Autodesk Inventor part; units mm, degrees
ref_plane "YZ Plane" through (0, 0, 0) normal (1, 0, 0) x (0, 1, 0)
ref_plane "XZ Plane" through (0, 0, 0) normal (0, 1, 0) x (-1, 0, 0)
ref_plane "XY Plane" through (0, 0, 0) normal (0, 0, 1) x (1, 0, 0)
sketch "Sketch1" plane through (0, 0, 0) normal (0, 1, 0) x (-1, 0, 0)
  circle A0 centre (0, 0) radius 30
  circle A1 centre (0, 0) radius 8.5
  dimension "d0" = 60
  dimension "d1" = 17
extrude "Extrusion1" add sketch "Sketch1" along normal blind 30
sketch "Sketch2" plane through (0, 30, 0) normal (0, 1, 0) x (1, 0, 0)
  circle A0 centre (0, 0) radius 21
  dimension "d4" = 42
extrude "Extrusion2" cut sketch "Sketch2" against normal blind 20
fillet "Fillet1" radius 2 1 edges at (30, 30, 0)
fillet "Fillet2" radius 0.5 1 edges at (-21, 30, 0)
shell "Shell2" thickness 1.5 removed faces 1 at (-22.4604, 0, -3.0712)
properties part number "FrontWheel"
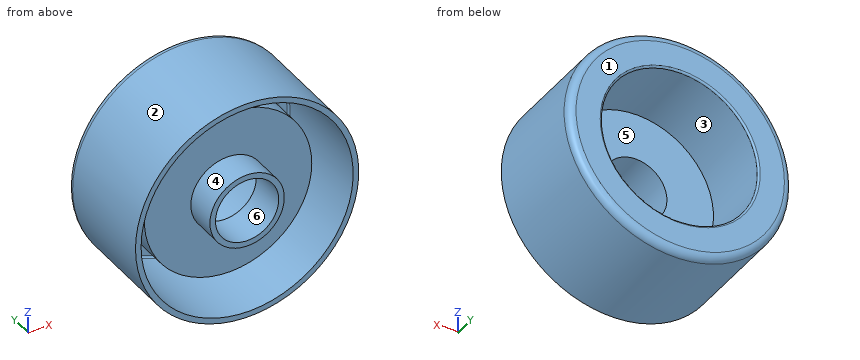
The listing builds one solid part. Answer for the finished solid, in the listing's coordinates (mm). Face numbers are marked on the shaded views. A direction names the side the tool comes from. Coordinates: 2 decimals unless noted, no trailing zeros. Order: outer loops, then holes, each group sorted by start corner. A loop starts at its lowest first (then second) coordinate and runs counter-clockwise, first axis right, second up. Notation, with made-up numbers: M -23.5,-4 L 14.5,-4 A25 cw 14.5,18 Z; hole C 6,-40 d10. An arc over 180 degrees is marked long. Use CSV: the item, a comma, the result in double quotes.
Q1. Determine the mould class of the marked faces 1, 2 and 3 for opening direction X: pulls with the +X half, pulls with the -X half, needs draft (parallel to the pull), parting line crosses it, or undercut.
Here are the results:
face 1,"needs draft"
face 2,"parting line crosses it"
face 3,"undercut"
Q2. Straight lines are drawn through the part: L1, parallel to Z at x = 0, y = 13; L2, parallel to Z at x = 5, y = 11.75; L3, parallel to X at y = 3.5, z = -1. For each, find the intervals that lie inside material, in ascending order.
Here are the results:
L1,"-30 to -28.5, -22.5 to -21, 21 to 22.5, 28.5 to 30"
L2,"-29.58 to -28.06, -21.94 to -20.4, 20.4 to 21.94, 28.06 to 29.58"
L3,"-29.98 to -28.48, -9.95 to -8.44, 8.44 to 9.95, 28.48 to 29.98"
Q3. A tool of negligible diameter and unlimited length cuts with its end or side. For the marked faces 4, 5 and 6, from which of +Z, -Z, +X, -X, +Y, -Y can it reach the whole face along a straight path? Write none if from no direction.
Here are the results:
face 4,"-Y"
face 5,"+Y"
face 6,"+Y, -Y"
Q4. Section C-C (y = 12.25) is taken. Determine the outline of the cut face in (x, z), then the cut area to 3 significant figures.
Here are the results:
outline,"C 0,0 d60; C 0,0 d45; hole C 0,0 d57; hole C 0,0 d42"
area,"481 mm2"
Q5. Given pin 1 Ø8 at (x, y) = (-15.5, 8.5) entering from -Z; pin 2 Ø8 at (y, z) = (22, -6) entering from -X; pin 3 Ø12 at (x, y) = (-0.5, 13) entering from +Z, each flat-ended and moving along its own axis, determine where each tip first touches the part or whether it passes through.
Here are the results:
pin 1,"z = -27.71"
pin 2,"x = -29.93"
pin 3,"z = 30"
